```python
from build123d import *

# Parameters (mm, degrees)
BOSS_EXTRUDE2_DEPTH = 40
SKETCH7_R           = 2.5
CUT_EXTRUDE1_DEPTH  = 61.804276165
SKETCH8_R           = 0.75
BOSS_EXTRUDE3_DEPTH = 5


with BuildPart() as part:
    # Sketch1 → Boss-Extrude2 (new body)
    with BuildSketch(Plane.XY):
        Polygon((-4.44e-06, 34.6), (4.99999556, 34.6), (14.99999556, -0.4), (19.99999556, -0.4), (19.99999556, -5.4), (19.99999556, -15.4), (-1.2662e-05, -15.4), (-10.00000444, -15.4), (-10.00000444, -5.4), (-4.44e-06, -5.4), (2.49999556, -5.4), (2.49999556, 1.6), (-4.44e-06, 1.6), align=None)
    extrude(amount=BOSS_EXTRUDE2_DEPTH)

    # Sketch7 → Cut-Extrude1 (cut, through all)
    with BuildSketch(Plane(origin=(19.99999556, 0, 0), x_dir=(0, 0, -1), z_dir=(1, 0, 0))):
        with Locations((-35, -10.4)):
            Circle(SKETCH7_R)
        with Locations((-5, -10.4)):
            Circle(SKETCH7_R)
    extrude(amount=-CUT_EXTRUDE1_DEPTH, mode=Mode.SUBTRACT)

    # Sketch8 → Boss-Extrude3 (add)
    with BuildSketch(Plane(origin=(0, -5.4, 0), x_dir=(1, 0, 0), z_dir=(0, 1, 0))):
        with Locations(Location((-5.00000444, -20, 0), (0, 0, 90))):
            Circle(SKETCH8_R)
    extrude(amount=BOSS_EXTRUDE3_DEPTH)


solid = part.part
```
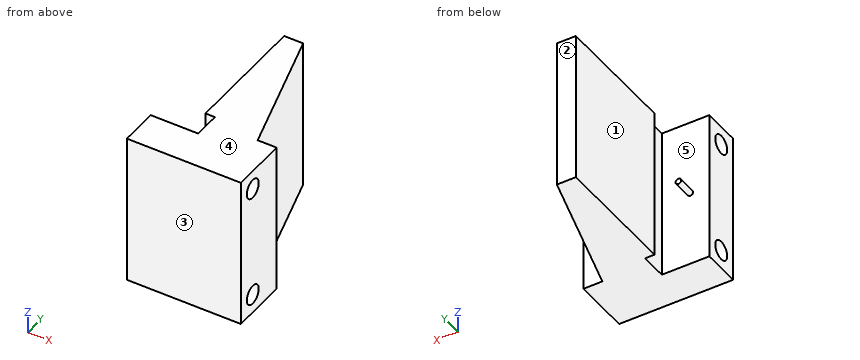
CAD build for the part. Positions are in the model's coordinates, mm. Face numbers are marked on the shaded views. A direction names the side the tool comes from. Round coordinates to 2 decimals unless told otherwise and drop trailing zeros. Loops run counter-clockwise (first coordinate to the right, second up) from the corner with the lowest first, then second, coordinate; pieces in that order, holes last. Notation, with made-up numbers: M 72,48 L 106,48 A20 ccw 106,56 Z; hole C 53.25,65 d2. An arc over 180 degrees is marked long. Use a Markdown table: item, result. Add a question column.
(1) Cut at D-D (z = 28). Give the cut face in (x, y).
(2) Which spindle directions (+Z, -Z, +X, -X, +Y, -Y) get a long thin tool onto all of the face, cutting with end or side? Do the marked faces 1 and 2. Say none if no direction does.
(3) Drill centre lines: line 1 (Y direction, x = -3, z = 35); line 2 (X direction, y = -3, z = 9.5); line 3 (Y direction, x = -4, z = 12). Where is each one in solid material? Low to high.
(4) Cut at A-A (z = 6.5). Give the cut face in (x, y), and give its area (4 significant figures).
(5) Cut at B-B (y = -10.4). Give the cut face in (x, z).
(6) Pull direction Y, two halves, no side cores. Call the marked faces 3, 4 and 5: +Y half, -Y half, draft (parallel to the pull), parting line (faces both ways), or undercut.
(7) Flat gauge pins, fed straight in: pin 1 (1.2 mm diameter, centred on x = -4.5, z = 20.5, fed in from +Y); pin 2 (4 mm diameter, centred on y = 17, z = 11, fed in from -X); pin 3 (6.5 mm diameter, centred on y = -10.4, z = 35, fed in from +X); pin 4 (4 mm diameter, centred on x = -7, z = 24.5, fed in from +Y). Where does each tip first touch, or does it go through?
(8) Cut at C-C (x = -1.5). Give the cut face in (y, z), and give its area (3 significant figures).
Geometry says:
| question | item | result |
|---|---|---|
| 1 | outline | M -10,-15.4 L 20,-15.4 L 20,-0.4 L 15,-0.4 L 5,34.6 L 0,34.6 L 0,1.6 L 2.5,1.6 L 2.5,-5.4 L -10,-5.4 Z |
| 2 | face 1 | +Z, -Z, -X, +Y |
| 2 | face 2 | +Z, -Z, +X, -X, +Y |
| 3 | line 1 | y = -15.4 to -12.9, -7.9 to -5.4 |
| 3 | line 2 | x = 2.5 to 20 |
| 3 | line 3 | y = -15.4 to -5.4 |
| 4 | outline | M -10,-15.4 L 20,-15.4 L 20,-12.4 L -10,-12.4 Z; M -10,-8.4 L 20,-8.4 L 20,-0.4 L 15,-0.4 L 5,34.6 L 0,34.6 L 0,1.6 L 2.5,1.6 L 2.5,-5.4 L -10,-5.4 Z |
| 4 | area | 612.5 mm² |
| 5 | outline | M -10,0 L 20,0 L 20,2.5 L -10,2.5 Z; M -10,7.5 L 20,7.5 L 20,32.5 L -10,32.5 Z; M -10,37.5 L 20,37.5 L 20,40 L -10,40 Z |
| 6 | face 3 | -Y half |
| 6 | face 4 | draft |
| 6 | face 5 | undercut |
| 7 | pin 1 | stops at y = -0.4 |
| 7 | pin 2 | stops at x = 0 |
| 7 | pin 3 | stops at x = 20 |
| 7 | pin 4 | stops at y = -5.4 |
| 8 | outline | M -15.4,0 L -5.4,0 L -5.4,40 L -15.4,40 Z; hole C -10.4,5 d5; hole C -10.4,35 d5 |
| 8 | area | 361 mm² |
